Drawing for the job (mm, zero at the part's lowest x, y, z). Coordinates: 2 decimals unless noted, no trailing zeros. Write each loop counter-clockwise with the first axis right and the second up, starting at its lowest first coordinate (ties: lowest second). Pieces come first, ordered by that corner, then holes. Notation, with made-up numbers: M 34,19 L 72,19 A30 cw 72,44 Z; hole C 81.5,5.5 d4. An arc over 180 degrees is marked long. Use a Markdown table: item, result. Add a question column.
Q1. Slice it at A-A on x = 25.4. Write the cut outline in (y, z).
Q2. Pin check, flat tip, straight feed: pin 1 Ø5 at (y, z) = (34.5, 6) entering from -X. Stop position of the tip, or through.
Q3. Wall check: L1, parallel to Y at x = 25.4, z = 12.5; L2, parallel to X at y = 38.1, z = 22; L3, parallel to Y at x = 25, z = 28. Give the ranges that are in metal, low to high. Write a range as from..to.
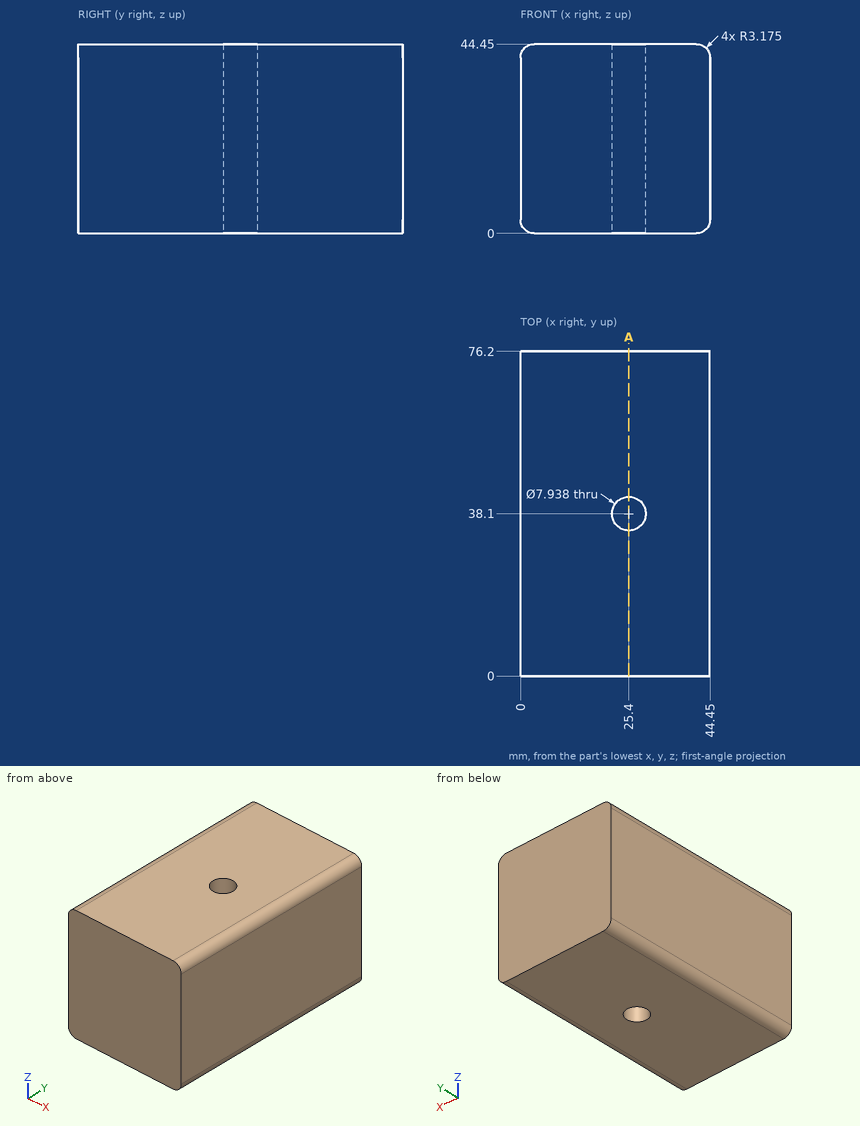
Recorded:
| question | item | result |
|---|---|---|
| 1 | outline | M 0,0 L 34.13,0 L 34.13,44.45 L 0,44.45 Z; M 42.07,0 L 76.2,0 L 76.2,44.45 L 42.07,44.45 Z |
| 2 | pin 1 | x = 0 |
| 3 | L1 | 0..34.13, 42.07..76.2 |
| 3 | L2 | 0..21.43, 29.37..44.45 |
| 3 | L3 | 0..34.15, 42.05..76.2 |
